Verification items for the finished model (mm, model axes). Coordinates: 2 decimals unless noted, no trailing zeros. Loops run counter-clockwise (first coordinate to the right, second up) from the corner with the lowest first, then second, coordinate; pieces in that order, holes last.
Q1. Sectioned sample at A-A (x = -143). Enter the section's corners in (y, z), then the cut area to 3 significant figures.
Q2. Sectioned sample at B-B (y = -2). Count the separate pieces of the cut face and the enclosed holes in it, then the cut area to 3 significant figures.
Q3. Material ranges on probe 1 along X at (y, z) = (-1.4, -28.75); probe 2 along Z at (x, y) = (18, -2.05); probe 3 along Z at (x, y) = (20, -0.95), recorded low to high.
Q4. Go/stop test with a flat-tipped pin: P1, Ø1.5, axis at x = 112, y = -0.5, coming from the -Z side. Record where the tip stops, or that it passes through.
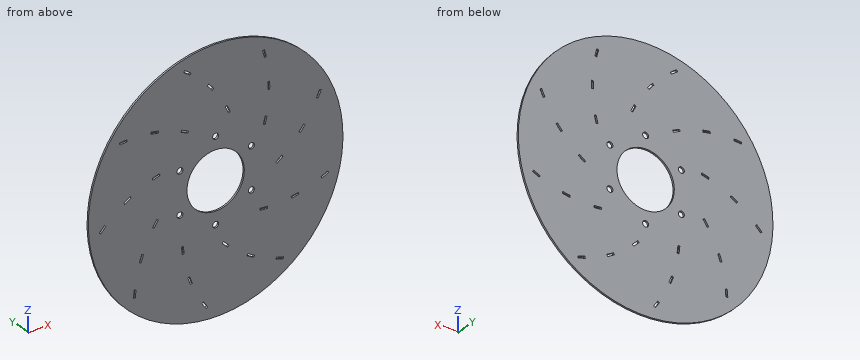
```python
from build123d import *

# Parameters (mm, degrees)
SKETCH2_R                = 177.5
SKETCH2_R_2              = 40
SKETCH2_R_3              = 4.15
BASE_FLANGE1_DEPTH       = 2.5
TAB_START                = -2.5
TAB_AND_SLOT_SLOT1_DEPTH = 2.5
CIRPATTERN1_COUNT        = 9


# Read off the part's stored shape, not the designer's step: Tab and Slot-Slot1
# Sheet-metal steps are written as plain solids
with BuildPart() as part:
    # Sketch2 → Base-Flange1 (new body)
    with BuildSketch(Plane(origin=(0, 0, 0), x_dir=(1, 0, 0), z_dir=(0, 1, 0))):
        with Locations(Location((0, 0, 0), (0, 0, 270))):
            Circle(SKETCH2_R)
        with Locations(Location((0, 0, 0), (0, 0, 270))):
            Circle(SKETCH2_R_2, mode=Mode.SUBTRACT)
        with Locations(Location((0, 57.5, 0), (0, 0, 270))):
            Circle(SKETCH2_R_3, mode=Mode.SUBTRACT)
        with Locations(Location((49.796460718, 28.75, 0), (0, 0, 270))):
            Circle(SKETCH2_R_3, mode=Mode.SUBTRACT)
        with Locations(Location((49.796460718, -28.75, 0), (0, 0, 270))):
            Circle(SKETCH2_R_3, mode=Mode.SUBTRACT)
        with Locations(Location((0, -57.5, 0), (0, 0, 270))):
            Circle(SKETCH2_R_3, mode=Mode.SUBTRACT)
        with Locations(Location((-49.796460718, -28.75, 0), (0, 0, 270))):
            Circle(SKETCH2_R_3, mode=Mode.SUBTRACT)
        with Locations(Location((-49.796460718, 28.75, 0), (0, 0, 270))):
            Circle(SKETCH2_R_3, mode=Mode.SUBTRACT)
    extrude(amount=-BASE_FLANGE1_DEPTH)

    # Tab and Slot-Slot1 outline → Tab and Slot-Slot1 (cut)
    with BuildSketch(Plane(origin=(0, 0, 0), x_dir=(1, 0, 0), z_dir=(0, 1, 0)).offset(TAB_START)):
        with BuildLine():
            Line((-19.35698036, 153.703677576), (-17.100043029, 152.221707173))
            ThreePointArc((-17.100043029, 152.221707173), (-14.185380107, 156.523975279), (-11.142966591, 160.736871053))
            Line((-11.142966591, 160.736871053), (-13.308830451, 162.349023691))
            ThreePointArc((-13.308830451, 162.349023691), (-16.397738089, 158.071706572), (-19.35698036, 153.703677576))
        make_face()
        with BuildLine():
            ThreePointArc((-36.160055897, 113.251731275), (-34.405862702, 118.143313538), (-32.505717981, 122.980070804))
            Line((-32.505717981, 122.980070804), (-35.004247803, 124.003472544))
            ThreePointArc((-35.004247803, 124.003472544), (-36.933420587, 119.092761343), (-38.714454271, 114.126403408))
            Line((-38.714454271, 114.126403408), (-36.160055897, 113.251731275))
        make_face()
        with BuildLine():
            ThreePointArc((-44.938772946, 70.767884474), (-44.45508819, 75.941937031), (-43.816406366, 81.09915104))
            Line((-43.816406366, 81.09915104), (-46.490871974, 81.469604956))
            ThreePointArc((-46.490871974, 81.469604956), (-47.139294904, 76.233543475), (-47.630397611, 70.980391064))
            Line((-47.630397611, 70.980391064), (-44.938772946, 70.767884474))
        make_face()
    tab_and_slot_slot1 = extrude(amount=TAB_AND_SLOT_SLOT1_DEPTH, mode=Mode.SUBTRACT)

    # CirPattern1: Tab and Slot-Slot1 ×9 about axis
    cirpattern1_axis = Axis((0, 0, 0), (0, 1, 0))
    for i in range(1, CIRPATTERN1_COUNT):
        add(tab_and_slot_slot1.rotate(cirpattern1_axis, i * 360 / CIRPATTERN1_COUNT), mode=Mode.SUBTRACT)


solid = part.part
```
Geometry check:
1. outline: (-2.5, -105.15) - (0, -105.15) - (0, 105.15) - (-2.5, 105.15) - close
1. area: 526 mm2
2. separate pieces: 1
2. enclosed holes: 34
2. area: 92,900 mm2
3. probe 1: x = -175.16 to -85.55, -82.3 to -53.95, -45.65 to -27.81, 27.81 to 45.65, 53.95 to 175.16
3. probe 2: z = -176.58 to -90.91, -89.78 to -35.72, 35.72 to 81.92, 88.21 to 176.58
3. probe 3: z = -176.37 to -34.64, 34.64 to 82.77, 84.04 to 176.37
4. P1: stops at z = -138.31
